The listing builds one solid part. Answer for the finished solid, in the listing's coordinates (mm). A direction names the side the tool comes from. Round coordinates to 2 decimals unless told otherwise and drop trailing zeros. Loops run counter-clockwise (first coordinate to the right, second up) from the corner with the lowest first, then second, coordinate; pieces in that order, holes last. Notation, with made-up numbers: (-25, -25) - (21, -25) arc R13 cw to (21, -5) - close; hole circle Ø1 at (49.25, 40). An arc over 180 degrees is marked (long way). Write item = value, one per line. Start each with the question number.
1) Section B-B, the plane y = 11.5 is taken. Determine the outline of the cut face in (x, z), and give its area (3 significant figures).
2) Straight lines are drawn through the part: line 1 along Z through (x, y) = (-21, -1.1); line 2 along Z through (x, y) = (27, -3.4); line 3 along Y through (x, z) = (-18, -12.5). For each, find the intervals that lie inside material, in ascending order.
3) A tool of negligible diameter and unlimited length cuts with its end or side. For faces 1 (the cylindrical face through (21, -2, 21)), 2 (the flat face through (15, 7, 10)), 3 (the flat face through (11, 7, 10)), 4 (the flat face through (13, 7, 15)), 5 (the flat face through (-13, 7, 5)), from which of +Z, -Z, +X, -X, +Y, -Y can it reach the whole face along a straight path? Write none if from no direction.
4) Section A-A, the plane x = 27 is taken. Determine the outline of the cut face in (y, z).
5) For a pull along Z with two mould halves and no side action, classify faces 6 (the flat face through (0, -2, -25)), 7 (the flat face through (-13, 15, 10)), 8 (the cylindrical face through (19.4, -2.5, -6.2)) as released by +Z, released by -Z, zero draft, split by the parting line, or undercut.
6) Section C-C, the plane x = -21 is taken. Determine the outline of the cut face in (y, z), and give its area (3 significant figures).
7) Given pin 1 Ø4.5 at (x, z) = (-21, -5) entering from +Y; pin 2 Ø3 at (x, z) = (21, -5) entering from +Y; pin 3 Ø8 at (y, z) = (5, 12.5) entering from +X; pin 4 Ø3 at (x, y) = (14, 7.5) entering from +Z, each flat-ended and moving along its own axis, determine where each tip first touches the part or whether it passes through.
8) Section D-D, the plane z = -17 is taken. Determine the outline of the cut face in (x, y).
from build123d import *

# Parameters (mm, degrees)
F0_W     = 70
F0_H     = 50
F0_R     = 4
F0_R_2   = 2
F1_DEPTH = 5
F2_R     = 4
F3_R     = 0.5
F4_W     = 4
F4_H     = 10
F5_DEPTH = 15


with BuildPart() as f1:
    # F0 (on Front) → F1 (new body)
    with BuildSketch(Plane.XZ):
        Rectangle(F0_W, F0_H)
        with Locations((-27, -17)):
            Circle(F0_R, mode=Mode.SUBTRACT)
        with Locations((-21, -5)):
            Circle(F0_R_2, mode=Mode.SUBTRACT)
        with Locations((27, -17)):
            Circle(F0_R, mode=Mode.SUBTRACT)
        with Locations((21, -5)):
            Circle(F0_R_2, mode=Mode.SUBTRACT)
        with Locations((-21, 19)):
            Circle(F0_R_2, mode=Mode.SUBTRACT)
        with Locations((21, 19)):
            Circle(F0_R_2, mode=Mode.SUBTRACT)
    extrude(amount=F1_DEPTH)

    # F2
    f2_edges = [f1.edges().sort_by_distance(p)[0] for p in [
        (35, -2.5, -25),
        (-35, -2.5, -25),
    ]]
    fillet(f2_edges, radius=F2_R)

    # F3
    f3_edges = [f1.edges().sort_by_distance(p)[0] for p in [
        (-31, -5, -17),
        (23, -5, -17),
        (-31, 0, -17),
        (23, 0, -17),
    ]]
    fillet(f3_edges, radius=F3_R)

    # F4 (on face) → F5 (join)
    with BuildSketch(Plane(origin=(0, 0, 0), x_dir=(-1, 0, 0), z_dir=(0, 1, 0))):
        with Locations((-13, 10)):
            Rectangle(F4_W, F4_H)
        with Locations((13, 10)):
            Rectangle(F4_W, F4_H)
    extrude(amount=F5_DEPTH)


solid = f1.part
Geometry check:
q1.outline = (-15, 5) - (-11, 5) - (-11, 15) - (-15, 15) - close; (11, 5) - (15, 5) - (15, 15) - (11, 15) - close
q1.area = 80.0 mm2
q2.line_1 = -25 to -7, -3 to 17, 21 to 25
q2.line_2 = -25 to -21, -13 to 25
q2.line_3 = -5 to 0
q3.face_1 = +Y, -Y
q3.face_2 = +Z, -Z, +X, +Y
q3.face_3 = +Z, -Z, +Y
q3.face_4 = +Z, +X, -X, +Y
q3.face_5 = -Z, +X, -X, +Y
q4.outline = (-5, -25) - (0, -25) - (0, -21.5) arc R0.5 ccw to (-0.5, -21) - (-4.5, -21) arc R0.5 ccw to (-5, -21.5) - close; (-5, -12.5) arc R0.5 ccw to (-4.5, -13) - (-0.5, -13) arc R0.5 ccw to (0, -12.5) - (0, 25) - (-5, 25) - close
q5.face_6 = released by -Z
q5.face_7 = zero draft
q5.face_8 = undercut
q6.outline = (-5, -25) - (0, -25) - (0, -7) - (-5, -7) - close; (-5, -3) - (0, -3) - (0, 17) - (-5, 17) - close; (-5, 21) - (0, 21) - (0, 25) - (-5, 25) - close
q6.area = 210 mm2
q7.pin_1 = 0
q7.pin_2 = through
q7.pin_3 = 15
q7.pin_4 = 15
q8.outline = (-35, -5) - (-31.5, -5) arc R0.5 ccw to (-31, -4.5) - (-31, -0.5) arc R0.5 ccw to (-31.5, 0) - (-35, 0) - close; (-23, -4.5) arc R0.5 ccw to (-22.5, -5) - (22.5, -5) arc R0.5 ccw to (23, -4.5) - (23, -0.5) arc R0.5 ccw to (22.5, 0) - (-22.5, 0) arc R0.5 ccw to (-23, -0.5) - close; (31, -4.5) arc R0.5 ccw to (31.5, -5) - (35, -5) - (35, 0) - (31.5, 0) arc R0.5 ccw to (31, -0.5) - close
